Geometry: final body of the model. Coordinates: model frame, mm. A direction names the side the tool comes from. Give positions to 0.01 mm unless a question says otherwise; leave off trailing zeros. Answer in a Markdown table with one row per item. Add a question column.
Item 1: Material intervals for probe 1 along Y at (x, z) = (96.5, 34), sorted ascending. Write a range as from..to.
Item 2: Access query for faces 4 (the flat face through (52, -42, 21)), 5 (the flat face through (35.75, -40, 9)). Directions: +Z, -Z, +X, -X, +Y, -Y. A direction counts if a zero-diameter tool reaches every point of the face in a straight line with its end or side. Return the directions, or none.
Item 3: Draft query along X for faces 1 (the flat face through (106, -21, 21)), 2 (the flat face through (0, -21, 21)), 3 (the flat face through (94, -37.5, 9)). Return one class per face: +X half, -X half, draft (parallel to the pull), parting line (faces both ways), or undercut.
```python
from build123d import *

# Parameters (mm, degrees)
ESQUISSE1_W             = 106
ESQUISSE1_H             = 42
BOSS_EXTRU_1_DEPTH      = 42
ESQUISSE2_W             = 10.5
ESQUISSE2_H             = 10.5
ENL_V_MAT_EXTRU_1_DEPTH = 4.5
CONG_1_R                = 0.5
CHANFREIN1_SIZE         = 0.5


with BuildPart() as part:
    # Esquisse1 → Boss.-Extru.1 (new body)
    with BuildSketch(Plane.XY):
        with Locations((53, -21)):
            Rectangle(ESQUISSE1_W, ESQUISSE1_H)
    extrude(amount=BOSS_EXTRU_1_DEPTH)

    # Esquisse2 → Enlèv. mat.-Extru.1 (cut)
    with BuildSketch(Plane.XZ.offset(42)):
        with Locations((65, 33)):
            Rectangle(ESQUISSE2_W, ESQUISSE2_H)
        with Locations((94, 9)):
            Rectangle(ESQUISSE2_W, ESQUISSE2_H)
        with Locations((94, 33)):
            Rectangle(ESQUISSE2_W, ESQUISSE2_H)
        with Locations((65, 9)):
            Rectangle(ESQUISSE2_W, ESQUISSE2_H)
    enl_v_mat_extru_1 = extrude(amount=-ENL_V_MAT_EXTRU_1_DEPTH, mode=Mode.SUBTRACT)

    # Congé1
    cong_1_edges = [part.edges().sort_by_distance(p)[0] for p in [
        (106, -21, 42),
        (53, 0, 42),
        (0, -21, 42),
        (53, 0, 0),
        (106, -21, 0),
        (53, -42, 0),
        (0, -21, 0),
        (53, -42, 42),
        (0, 0, 21),
        (106, 0, 21),
        (106, -42, 21),
        (0, -42, 21),
    ]]
    fillet(cong_1_edges, radius=CONG_1_R)

    # Symétrie1: Enlèv. mat.-Extru.1 across plane
    add(enl_v_mat_extru_1.mirror(Plane(origin=(53, 0, 0), x_dir=(0, 0, 1), z_dir=(1, 0, 0))), mode=Mode.SUBTRACT)

    # Chanfrein1
    chanfrein1_edges = [part.edges().sort_by_distance(p)[0] for p in [
        (46.25, -42, 33),
        (41, -42, 27.75),
        (35.75, -42, 33),
        (41, -42, 38.25),
        (46.25, -42, 9),
        (41, -42, 3.75),
        (35.75, -42, 9),
        (41, -42, 14.25),
        (17.25, -42, 9),
        (12, -42, 3.75),
        (6.75, -42, 9),
        (12, -42, 14.25),
        (17.25, -42, 33),
        (12, -42, 27.75),
        (6.75, -42, 33),
        (12, -42, 38.25),
        (59.75, -42, 33),
        (65, -42, 27.75),
        (70.25, -42, 33),
        (65, -42, 38.25),
        (59.75, -42, 9),
        (65, -42, 3.75),
        (70.25, -42, 9),
        (65, -42, 14.25),
        (88.75, -42, 9),
        (94, -42, 3.75),
        (99.25, -42, 9),
        (94, -42, 14.25),
        (88.75, -42, 33),
        (94, -42, 27.75),
        (99.25, -42, 33),
        (94, -42, 38.25),
    ]]
    chamfer(chanfrein1_edges, length=CHANFREIN1_SIZE)


solid = part.part
```
Findings below:
| question | item | result |
|---|---|---|
| 1 | probe 1 | y = -37.5..0 |
| 2 | face 4 | +Z, -Z, +X, -X, -Y |
| 2 | face 5 | -Y |
| 3 | face 1 | +X half |
| 3 | face 2 | -X half |
| 3 | face 3 | undercut |
